```python
from build123d import *

# Parameters (mm, degrees)
SKETCH15_R          = 3.3
SKETCH15_R_2        = 2.5
SKETCH15_R_3        = 52.3875
SKETCH15_R_4        = 4.5
SKETCH15_R_5        = 27.4955
BOSS_EXTRUDE1_DEPTH = 9.525
PROFILE_DEPTH       = 804.13111067
PROF_FILLET_R       = 12.7
CUT_EXTRUDE2_DEPTH  = 804.13111067
FILLET2_R           = 6.35
CUT_EXTRUDE4_DEPTH  = 804.13111067
FILLET5_R           = 6.35


with BuildPart() as part:
    # Sketch15 → Boss-Extrude1 (new body)
    with BuildSketch(Plane(origin=(0, 0, 0), x_dir=(-1, 0, 0), z_dir=(0, 0, 1))):
        with BuildLine():
            ThreePointArc((-776.492771968, 151.978917225), (-781.907485254, 150.230614898), (-784.225, 145.034))
            Line((-784.225, 145.034), (-784.225, 0))
            ThreePointArc((-784.225, 0), (-782.179140867, -4.939140867), (-777.24, -6.985))
            Line((-777.24, -6.985), (-548.64, -6.985))
            ThreePointArc((-548.64, -6.985), (-545.651186694, -6.313257481), (-543.237237519, -4.427231931))
            Line((-543.237237519, -4.427231931), (-459.418508663, 97.860764379))
            ThreePointArc((-459.418508663, 97.860764379), (-449.426249212, 133.212914363), (-468.520845097, 164.597881552))
            ThreePointArc((-468.520845097, 164.597881552), (-470.201009111, 165.051242365), (-471.778645707, 164.316701751))
            Line((-471.778645707, 164.316701751), (-477.043529325, 159.051818133))
            ThreePointArc((-477.043529325, 159.051818133), (-484.127165713, 157.642795249), (-488.139723403, 163.648012211))
            Line((-488.139723403, 163.648012211), (-488.139723403, 170.220745001))
            ThreePointArc((-488.139723403, 170.220745001), (-488.796888696, 171.925600851), (-490.428332433, 172.748273949))
            ThreePointArc((-490.428332433, 172.748273949), (-494.978508993, 172.974), (-499.528685552, 172.748273949))
            ThreePointArc((-499.528685552, 172.748273949), (-501.160129289, 171.925600851), (-501.817294582, 170.220745001))
            Line((-501.817294582, 170.220745001), (-501.817294582, 163.648012211))
            ThreePointArc((-501.817294582, 163.648012211), (-508.317294582, 157.148012211), (-514.817294582, 163.648012211))
            Line((-514.817294582, 163.648012211), (-514.817294582, 164.225022653))
            ThreePointArc((-514.817294582, 164.225022653), (-516.106794745, 166.435870942), (-518.665995494, 166.401924563))
            Line((-518.665995494, 166.401924563), (-660.126842441, 139.458698233))
            Line((-660.126842441, 139.458698233), (-776.492771968, 151.978917225))
        make_face()
        with Locations((-777.24, 0)):
            Circle(SKETCH15_R, mode=Mode.SUBTRACT)
        with Locations((-709.220726776, 39.660663218)):
            Circle(SKETCH15_R_2, mode=Mode.SUBTRACT)
        with Locations((-666.75, 20.751477371)):
            Circle(SKETCH15_R_2, mode=Mode.SUBTRACT)
        with Locations((-624.279273224, 39.660663218)):
            Circle(SKETCH15_R_2, mode=Mode.SUBTRACT)
        with Locations((-666.75, 77.901477371)):
            Circle(SKETCH15_R_3, mode=Mode.SUBTRACT)
        with Locations((-548.64, 0)):
            Circle(SKETCH15_R, mode=Mode.SUBTRACT)
        with Locations((-723.58692632, 83.875279047)):
            Circle(SKETCH15_R_2, mode=Mode.SUBTRACT)
        with Locations((-709.220726776, 116.142291524)):
            Circle(SKETCH15_R_2, mode=Mode.SUBTRACT)
        with Locations((-628.509185847, 120.372204147)):
            Circle(SKETCH15_R_2, mode=Mode.SUBTRACT)
        with Locations((-777.24, 145.034)):
            Circle(SKETCH15_R, mode=Mode.SUBTRACT)
        with Locations((-666.75, 135.051477371)):
            Circle(SKETCH15_R_2, mode=Mode.SUBTRACT)
        with Locations((-609.91307368, 83.875279047)):
            Circle(SKETCH15_R_2, mode=Mode.SUBTRACT)
        with Locations((-508.317294582, 90.351987789)):
            Circle(SKETCH15_R_4, mode=Mode.SUBTRACT)
        with Locations((-481.639723403, 90.351987789)):
            Circle(SKETCH15_R_4, mode=Mode.SUBTRACT)
        with Locations((-528.75349974, 107.5)):
            Circle(SKETCH15_R_4, mode=Mode.SUBTRACT)
        with Locations((-494.978508993, 127)):
            Circle(SKETCH15_R_5, mode=Mode.SUBTRACT)
        with Locations((-461.203518245, 107.5)):
            Circle(SKETCH15_R_4, mode=Mode.SUBTRACT)
        with Locations((-533.38601136, 133.772278929)):
            Circle(SKETCH15_R_4, mode=Mode.SUBTRACT)
        with Locations((-456.571006625, 133.772278929)):
            Circle(SKETCH15_R_4, mode=Mode.SUBTRACT)
        with Locations((-520.04722577, 156.875733282)):
            Circle(SKETCH15_R_4, mode=Mode.SUBTRACT)
        with Locations((-494.978508993, 166)):
            Circle(SKETCH15_R_4, mode=Mode.SUBTRACT)
        with Locations((-469.909792215, 156.875733282)):
            Circle(SKETCH15_R_4, mode=Mode.SUBTRACT)
    extrude(amount=BOSS_EXTRUDE1_DEPTH)

    # Sketch18 → Profile (cut, through all)
    with BuildSketch(Plane.XY.offset(9.525)):
        with BuildLine():
            Line((560.237930497, 5.174747161), (656.843849148, -10.682497906))
            Line((656.843849148, -10.682497906), (765.728355379, 5.363957318))
            ThreePointArc((765.728355379, 5.363957318), (766.151220409, 6.191039265), (766.633408889, 6.985))
            Line((766.633408889, 6.985), (559.246591111, 6.985))
            ThreePointArc((559.246591111, 6.985), (559.779095511, 6.10004518), (560.237930497, 5.174747161))
        make_face()
        with BuildLine():
            Line((549.771402717, 6.892760905), (560.237930497, 5.174747161))
            ThreePointArc((560.237930497, 5.174747161), (559.779095511, 6.10004518), (559.246591111, 6.985))
            Line((559.246591111, 6.985), (548.64, 6.985))
            ThreePointArc((548.64, 6.985), (549.207578223, 6.961902036), (549.771402717, 6.892760905))
        make_face()
        with BuildLine():
            ThreePointArc((766.633408889, 6.985), (766.151220409, 6.191039265), (765.728355379, 5.363957318))
            Line((765.728355379, 5.363957318), (776.22161066, 6.910362375))
            ThreePointArc((776.22161066, 6.910362375), (776.729439616, 6.966315604), (777.24, 6.985))
            Line((777.24, 6.985), (766.633408889, 6.985))
        make_face()
        with BuildLine():
            Line((776.542475038, -12.680830372), (734.216175486, -69.849260886))
            Line((734.216175486, -69.849260886), (783.003068504, -141.087195416))
            ThreePointArc((783.003068504, -141.087195416), (783.91252795, -142.968183999), (784.225, -145.034))
            Line((784.225, -145.034), (784.225, -10.606591111))
            ThreePointArc((784.225, -10.606591111), (780.550393136, -12.260966409), (776.542475038, -12.680830372))
        make_face()
        with BuildLine():
            Line((782.853818423, -4.156352694), (776.542475038, -12.680830372))
            ThreePointArc((776.542475038, -12.680830372), (780.550393136, -12.260966409), (784.225, -10.606591111))
            Line((784.225, -10.606591111), (784.225, 0))
            ThreePointArc((784.225, 0), (783.873353099, -2.188344502), (782.853818423, -4.156352694))
        make_face()
    extrude(amount=-PROFILE_DEPTH, mode=Mode.SUBTRACT)

    # Prof Fillet
    prof_fillet_edges = [part.edges().sort_by_distance(p)[0] for p in [
        (734.216175486, -69.849260886, 4.7625),
        (656.843849148, -10.682497906, 4.7625),
        (660.126842441, -139.458698233, 4.7625),
    ]]
    fillet(prof_fillet_edges, radius=PROF_FILLET_R)

    # Sketch19 → Cut-Extrude2 (cut, through all)
    with BuildSketch(Plane.XY.offset(9.525)):
        with BuildLine():
            Line((732.946816776, -56.623554423), (772.979141054, -2.553504053))
            Line((772.979141054, -2.553504053), (694.45302227, -14.12600314))
            ThreePointArc((694.45302227, -14.12600314), (718.284506978, -31.22211205), (732.946816776, -56.623554423))
        make_face()
        with BuildLine():
            Line((735.318467656, -89.439839453), (772.613524345, -143.897556318))
            Line((772.613524345, -143.897556318), (704.133403657, -136.529539656))
            ThreePointArc((704.133403657, -136.529539656), (724.722491105, -116.293648856), (735.318467656, -89.439839453))
        make_face()
    extrude(amount=-CUT_EXTRUDE2_DEPTH, mode=Mode.SUBTRACT)

    # Fillet2
    fillet2_edges = [part.edges().sort_by_distance(p)[0] for p in [
        (735.318467656, -89.439839453, 4.7625),
        (772.613524345, -143.897556318, 4.7625),
        (704.133403657, -136.529539656, 4.7625),
        (772.979141054, -2.553504053, 4.7625),
        (732.946816776, -56.623554423, 4.7625),
        (694.45302227, -14.12600314, 4.7625),
    ]]
    fillet(fillet2_edges, radius=FILLET2_R)

    # Sketch22 → Cut-Extrude4 (cut, through all)
    with BuildSketch(Plane.XY.offset(9.525)):
        with BuildLine():
            Line((625.959276135, -18.482944043), (563.09944586, -8.164904037))
            Line((563.09944586, -8.164904037), (540.883041369, -18.482944043))
            Line((540.883041369, -18.482944043), (505.79558687, -61.301839836))
            Line((505.79558687, -61.301839836), (596.214449629, -63.096701449))
            ThreePointArc((596.214449629, -63.096701449), (606.783495422, -37.920687172), (625.959276135, -18.482944043))
        make_face()
        with BuildLine():
            Line((621.388723544, -133.908618474), (542.982722013, -148.842154434))
            Line((542.982722013, -148.842154434), (594.94086334, -84.057218462))
            ThreePointArc((594.94086334, -84.057218462), (603.082763934, -111.679107661), (621.388723544, -133.908618474))
        make_face()
        with BuildLine():
            Line((502.723422183, -71.402857307), (590.665799743, -73.148559395))
            Line((590.665799743, -73.148559395), (550.94559886, -122.674400877))
            ThreePointArc((550.94559886, -122.674400877), (535.868576594, -88.541862661), (502.723422183, -71.402857307))
        make_face()
    extrude(amount=-CUT_EXTRUDE4_DEPTH, mode=Mode.SUBTRACT)

    # Fillet5
    fillet5_edges = [part.edges().sort_by_distance(p)[0] for p in [
        (540.883041369, -18.482944043, 4.7625),
        (563.09944586, -8.164904037, 4.7625),
        (505.79558687, -61.301839836, 4.7625),
        (596.214449629, -63.096701449, 4.7625),
        (625.959276135, -18.482944043, 4.7625),
        (502.723422183, -71.402857307, 4.7625),
        (590.665799743, -73.148559395, 4.7625),
        (550.94559886, -122.674400877, 4.7625),
        (621.388723544, -133.908618474, 4.7625),
        (542.982722013, -148.842154434, 4.7625),
        (594.94086334, -84.057218462, 4.7625),
    ]]
    fillet(fillet5_edges, radius=FILLET5_R)


solid = part.part
```
Verification items for the finished model (mm, model axes). A direction names the side the tool comes from. Give positions to 0.01 mm unless a question says otherwise; leave off trailing zeros. Order: outer loops, then holes, each group sorted by start corner. A loop starts at its lowest first (then second) coordinate and runs counter-clockwise, first axis right, second up. Notation, with made-up numbers: (53, -33) -> (101, -33) arc R12 cw to (101, -10) -> close; hole circle Ø1 at (87.5, 79.5). An arc over 180 degrees is marked (long way). One line per item, written item: value.
(1) Draft check along X on faces 3 (the face through (619, -104, 9.525)), 4 (the face through (737.106, -70.013, 4.696)), 5 (the face through (508.17, -157.15, 4.7)). Enter one of: pulls with the +X half, pulls with the -X half, needs draft (parallel to the pull), parting line crosses it, or undercut.
Final values:
face 3: needs draft
face 4: pulls with the +X half
face 5: undercut
(2) Sectioned sample at A-A on y = -54.5. Record the cut outline in (x, z) (3 decimals), then the cut area to 3 significant figures.
Final values:
outline: (494.95, 0) -> (512.685, 0) -> (512.685, 9.525) -> (494.95, 9.525) -> close; (598.582, 0) -> (619.88, 0) -> (619.88, 9.525) -> (598.582, 9.525) -> close; (713.62, 0) -> (745.58, 0) -> (745.58, 9.525) -> (713.62, 9.525) -> close
area: 676 mm^2
(3) Tool access check on faces 1 (the face through (714.076, -133.862, 4.696)), 2 (the face through (718.448, -145.734, 4.696)). Record the directions out of +Z, -Z, +X, -X, +Y, -Y that give a thin tool (end or side, any length) a straight path to the whole face; none if there is none.
Final values:
face 1: +Z, -Z
face 2: +Z, -Z, -Y
(4) Scan lines: line 1 along Y through (x, z) = (546.5, 4.75); line 2 along Y through (x, z) = (577, 3.5); line 3 along Y through (x, z) = (514, 5.5). Record each from-to range of solid material in increasing order. Write a range as [from, to].
Final values:
line 1: [-161.1, -104.72], [-72.27, -62.11], [-15.87, -2.51], [2.51, 6.65]
line 2: [-155.29, -142.36], [-106.43, -90.19], [-72.88, -62.72], [-10.45, 2.42]
line 3: [-160.49, -146.85], [-107.15, -59.13], [-51.29, -31.25]
(5) Sectioned sample at B-B on x = 636.5. Record the cut outline in (y, z) (3 decimals).
Final values:
outline: (-143.959, 0) -> (-120.673, 0) -> (-120.673, 9.525) -> (-143.959, 9.525) -> close; (-35.13, 0) -> (-7.343, 0) -> (-7.343, 9.525) -> (-35.13, 9.525) -> close
(6) Sectioned sample at C-C on z = 2.5. Count the separate pieces of the cut face and the enclosed holes in it, then the cut area to 3 significant figures.
Final values:
separate pieces: 1
enclosed holes: 27
area: 20,100 mm^2
(7) Gauge pin test, flat ends, axial feed: pin 1 (5.5 mm diameter, centred on x = 777.24, y = 0, fed in from +Z); pin 2 (3 mm diameter, centred on x = 670, z = 3, fed in from -Y); pin 3 (0.5 mm diameter, centred on y = -164, z = 6.5, fed in from -X); pin 4 (1.5 mm diameter, centred on y = -43, z = 8.5, fed in from +X). Record the tip position at first contact, or that the pin passes through.
Final values:
pin 1: through
pin 2: y = -140.68
pin 3: x = 467.36
pin 4: x = 754.65
